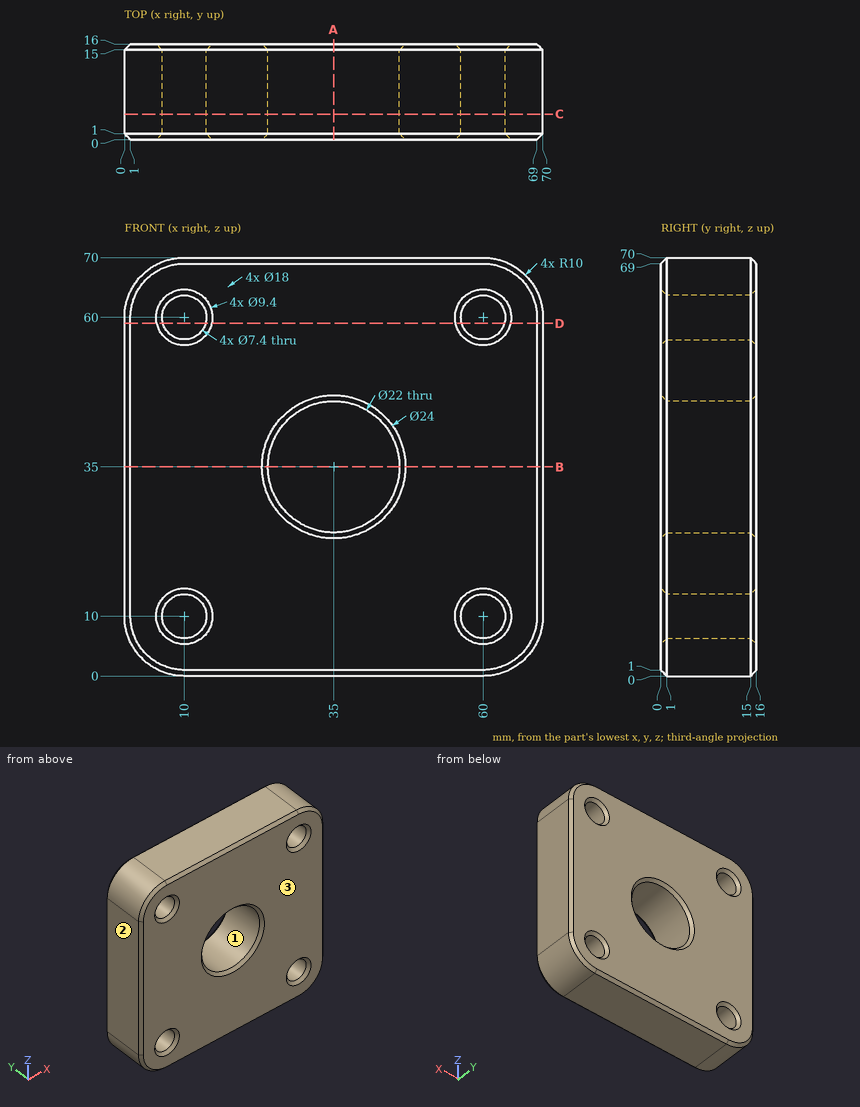
Verification items for this drawing (mm, ordinates from the low corner). Coordinates: 2 decimals unless noted, no trailing zeros. Write each loop counter-clockwise with the first axis right and the second up, starting at its lowest first coordinate (ties: lowest second). Pieces come first, ordered by that corner, then holes. Notation, with made-up numbers: M 88,28.5 L 119,28.5 A9 ccw 119,39.5 Z; hole C 76,38.25 d11. An arc over 180 degrees is marked long. One line per item, written item: value. Start each with the question number.
(1) Release check for a two-part mould opening along X. For the marked faces 1, 2 and 3 record: released by +X, released by -X, zero draft, split by the parting line, or undercut.
(2) Depth check by flat-ended pin: pin 1 (6.5 mm diameter, centred on x = 10, z = 10, fed in from -Y). Enter the tip coordinate at first touch or a pass-through.
(3) Scan lines: line 1 along X through (y, z) = (11.5, 60); line 2 along Z through (x, y) = (61.5, 1.5); line 3 along Z through (x, y) = (7, 11). Record each from-to range of solid material in increasing order. Write a range as [from, to].
(4) Sectioned sample at A-A, the plane x = 35. Enter the section's corners in (y, z), and give its area (3 significant figures).
(5) Sectioned sample at B-B, the plane z = 35. Enter the section's corners in (x, y), and give its area (3 significant figures).
(6) Sectioned sample at D-D, the plane z = 59. State how many separate pieces and enclosed holes the cut face has, and give its area (3 significant figures).
(7) Sectioned sample at C-C, the plane y = 4.25. Enter the section's corners in (x, z).
Filled sheet:
1. face 1: undercut
1. face 2: released by -X
1. face 3: zero draft
2. pin 1: through
3. line 1: [0, 6.3], [13.7, 56.3], [63.7, 70]
3. line 2: [0.11, 6.62], [13.38, 56.62], [63.38, 69.89]
3. line 3: [0.46, 7.83], [12.17, 57.83], [62.17, 69.54]
4. outline: M 0,1 L 1,0 L 15,0 L 16,1 L 16,23 L 15,24 L 1,24 L 0,23 Z; M 0,47 L 1,46 L 15,46 L 16,47 L 16,69 L 15,70 L 1,70 L 0,69 Z
4. area: 764 mm²
5. outline: M 0,1 L 1,0 L 23,0 L 24,1 L 24,15 L 23,16 L 1,16 L 0,15 Z; M 46,1 L 47,0 L 69,0 L 70,1 L 70,15 L 69,16 L 47,16 L 46,15 Z
5. area: 764 mm²
6. separate pieces: 3
6. enclosed holes: 0
6. area: 886 mm²
7. outline: M 0,10 A10 ccw 10,0 L 60,0 A10 ccw 70,10 L 70,60 A10 ccw 60,70 L 10,70 A10 ccw 0,60 Z; hole C 10,10 d7.4; hole C 10,60 d7.4; hole C 35,35 d22; hole C 60,10 d7.4; hole C 60,60 d7.4
